Autodesk Inventor part; units mm, degrees
ref_plane "YZ Plane" through (0, 0, 0) normal (1, 0, 0) x (0, 1, 0)
ref_plane "XZ Plane" through (0, 0, 0) normal (0, 1, 0) x (-1, 0, 0)
ref_plane "XY Plane" through (0, 0, 0) normal (0, 0, 1) x (1, 0, 0)
sketch "Esboço1" plane through (0, 0, 0) normal (0, 1, 0) x (-1, 0, 0)
  line L0 (20, -40) -> (-20, -40)
  line L1 (-20, -40) -> (-20, 40)
  line L2 (-20, 40) -> (20, 40)
  line L3 (20, 40) -> (20, -40)
  line L4 (20, -40) -> (-20, 40) construction
  line L5 (-20, -40) -> (20, 40) construction
  point P0 (0, 0)
  dimension "d0" = 40
  dimension "d1" = 80
extrude "Extrusão1" add sketch "Esboço1" along normal blind 80
sketch "Esboço2" plane through (20, 0, 40) normal (1, 0, 0) x (0, 0, -1)
  line L0 (0, 80) -> (20, 80)
  line L1 (20, 80) -> (20, 40)
  line L2 (20, 40) -> (0, 40)
  line L3 (0, 40) -> (0, 80)
  line L4 (80, 80) -> (60, 80)
  line L5 (60, 80) -> (60, 40)
  line L6 (60, 40) -> (80, 40)
  line L7 (80, 40) -> (80, 80)
  line L8 (0, 0) -> (80, 0)
  point P0 (40, 0)
  dimension "d4" = 20
  dimension "d5" = 20
  dimension "d6" = 40
extrude "Extrusão2" cut sketch "Esboço2" against normal through all contours L0 L1 L2 L3
extrude "Extrusão3" cut sketch "Esboço2" against normal through all contours L7 L6 L5 L4
fillet "Arredondamento1" radius 20 2 edges at (0, 80, 20) (0, 80, -20)
sketch "Esboço3" plane through (20, 0, 40) normal (1, 0, 0) x (0, 0, -1)
  arc A0 (60, 60) -> (20, 60) centre (40, 60) ccw
  point P0 (40, 0)
hole "Furo1" at (20, 60, 0) direction (-1, 0, 0) diameter 20 end through all
sketch "Esboço4" plane through (20, 40, 40) normal (0, 1, 0) x (1, 0, 0)
  line L0 (-35, 0) -> (-35, 5)
  line L1 (-35, 5) -> (-20, 13)
  line L2 (-20, 13) -> (-5, 5)
  line L3 (-5, 5) -> (-5, 0)
  line L4 (-40, 0) -> (-40, 20)
  line L5 (0, 0) -> (-40, 0)
  point P0 (-20, 40)
  dimension "d19" = 5
  dimension "d20" = 30
  dimension "d21" = 20
  dimension "d22" = 13
  dimension "d23" = 5
extrude "Extrusão4" cut sketch "Esboço4" against normal through all
mirror "Espelhar1" about plane through (0, 0, 0) normal (0, 0, 1) of "Extrusão4"
sketch "Esboço6" plane through (20, 0, 40) normal (1, 0, 0) x (0, 0, -1)
  line L0 (20, 20) -> (60, 20)
  line L1 (60, 20) -> (60, 0)
  line L2 (60, 0) -> (20, 0)
  line L3 (20, 0) -> (20, 20)
  line L4 (0, 0) -> (80, 0)
  point P0 (40, 0)
  point P1 (40, 0)
  dimension "d26" = 40
  dimension "d27" = 20
extrude "Extrusão5" cut sketch "Esboço6" against normal through all
fillet "Arredondamento2" radius 5 2 edges at (0, 20, -20) (0, 20, 20)
properties part number "3D Model"
The listing builds one solid part. Answer for the finished solid, in the listing's coordinates (mm). A direction names the side the tool comes from. Give positions to 0.01 mm unless a question says otherwise; leave off trailing zeros. Loops run counter-clockwise (first coordinate to the right, second up) from the corner with the lowest first, then second, coordinate; pieces in that order, holes last. Notation, with made-up numbers: M 49,33.25 L 87,33.25 A33 cw 87,70.25 Z; hole C 4,17.5 d11. An arc over 180 degrees is marked long. One line per item, written item: value.
Q1. A cutting plane is placed at D-D on y = 51.5. Determine the outline of the cut face in (x, z), then the cut area to 3 significant figures.
Working result:
outline: M -20,-20 L 20,-20 L 20,-5.27 L -20,-5.27 Z; M -20,5.27 L 20,5.27 L 20,20 L -20,20 Z
area: 1,180 mm^2
Q2. For faces 1 (the face through (0, 18, 19)), 2 (the face through (15, 20, -38)), 3 (the face through (0, 40, -25)), determine the directions among +Z, -Z, +X, -X, +Y, -Y from which every point of the face is accessible in a straight line to the end or side of a thin tool.
Working result:
face 1: +X, -X, -Y
face 2: -Z, +Y, -Y
face 3: -Z, +X, -X, +Y
Q3. A cutting plane is placed at A-A on y = 9. Determine the outline of the cut face in (x, z), then the cut area to 3 significant figures.
Working result:
outline: M -20,-40 L -15,-40 L -15,-35 L 0,-27 L 15,-35 L 15,-40 L 20,-40 L 20,-20 L -20,-20 Z; M -20,20 L 20,20 L 20,40 L 15,40 L 15,35 L 0,27 L -15,35 L -15,40 L -20,40 Z
area: 1,060 mm^2
Q4. Find the intervals of material crossed by line 1 (Z direction, x = -8, y = 60); line 2 (Y direction, x = -6, z = 0); line 3 (Z direction, x = 10, y = 43), in increasing order. Write a range as from..to.
Working result:
line 1: z = -20..-10, 10..20
line 2: y = 20..50, 70..80
line 3: z = -20..20
Q5. Determine the mould class of faces 4 (the face through (-15, 20, -37)), 5 (the face through (20, 39, -1)), 6 (the face through (17, 20, -40)) for opening direction X: +X half, -X half, draft (parallel to the pull), parting line (faces both ways), or undercut.
Working result:
face 4: undercut
face 5: +X half
face 6: draft
Q6. Flat-ended cylindrical pins translate along their axes: P1, Ø7.5, axis at x = 0, y = 5, coming from the +Z side; P2, Ø18, axis at y = 60, z = 0, coming from the +X side; P3, Ø10, axis at x = -4, z = -34, coming from the +Y side; P4, Ø22, axis at x = -9.5, y = 51.5, coming from the +Z side. Find the tip coordinate at first contact, or state that the pin passes through.
Working result:
P1: stops at z = 29
P2: passes through
P3: stops at y = 40
P4: stops at z = 20
Q7. A cutting plane is placed at C-C on z = -8. Determine the outline of the cut face in (x, y).
Working result:
outline: M -20,20 L 20,20 L 20,54 L -20,54 Z; M -20,66 L 20,66 L 20,78.33 L -20,78.33 Z
